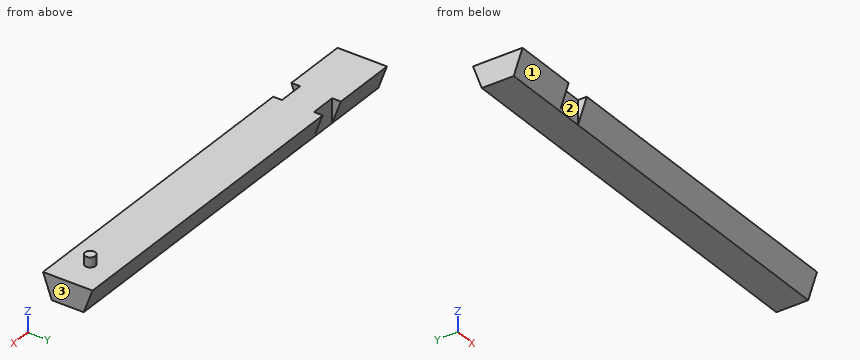
```python
from build123d import *

# Parameters (mm, degrees)
F1_DEPTH  = 203
F2_R      = 2.5
F3_DEPTH  = 10
F4_W      = 12.5
F4_H      = 4.258452
F5_DEPTH  = 11.701
F3_FACE_R = 2.5
F6_DEPTH  = 14.7


with BuildPart() as f1:
    # F0 (on Right) → F1 (new body)
    with BuildSketch(Plane.YZ):
        Polygon((-12, 11.7), (-7.741548, 0), (0, 0), (0, 11.7), align=None)
        Polygon((0, 11.7), (0, 0), (7.741548, 0), (12, 11.7), align=None)
    extrude(amount=F1_DEPTH)

    # F2 (on face) → F3 (cut)
    with BuildSketch(Plane.XY.offset(11.7)):
        with Locations((187.5, 0)):
            Circle(F2_R)
    extrude(amount=-F3_DEPTH, mode=Mode.SUBTRACT)

    # F4 (on face) → F5 (cut, through all)
    with BuildSketch(Plane.XY.offset(11.7)):
        with Locations((38.05, 9.870774)):
            Rectangle(F4_W, F4_H)
        with Locations((38.05, -9.870774)):
            Rectangle(F4_W, F4_H)
    extrude(amount=-F5_DEPTH, mode=Mode.SUBTRACT)

    # F3_face (on face) → F6 (join)
    with BuildSketch(Plane(origin=(187.5, 0, 1.7), x_dir=(1, 0, 0), z_dir=(0, 0, 1))):
        Circle(F3_FACE_R)
    extrude(amount=F6_DEPTH)


solid = f1.part
```
Source: CAD feature listing. Evaluate the final solid. Frame: model axes, mm. Face numbers are marked on the shaded views. Round coordinates to 2 decimals unless told otherwise and drop trailing zeros. Loops run counter-clockwise (first coordinate to the right, second up) from the corner with the lowest first, then second, coordinate; pieces in that order, holes last.
(1) Section query C-C (z = 7.75). Output: boundary loops of the cut face in (x, y).
From the geometry:
outline: (0, -10.56) - (31.8, -10.56) - (31.8, -7.74) - (44.3, -7.74) - (44.3, -10.56) - (203, -10.56) - (203, 10.56) - (44.3, 10.56) - (44.3, 7.74) - (31.8, 7.74) - (31.8, 10.56) - (0, 10.56) - close
(2) Section query B-B (y = 0). Output: boundary loops of the cut face in (x, z), and give its area (3 significant figures).
From the geometry:
outline: (0, 0) - (203, 0) - (203, 11.7) - (190, 11.7) - (190, 16.4) - (185, 16.4) - (185, 11.7) - (0, 11.7) - close
area: 2,400 mm2
(3) Material intervals for probe 1 along X at (y, z) = (8, 9.25); probe 2 along Y at (x, z) = (37, 4.75); probe 3 along Z at (x, y) = (14, -2), sorted ascending.
From the geometry:
probe 1: x = 0 to 31.8, 44.3 to 203
probe 2: y = -7.74 to 7.74
probe 3: z = 0 to 11.7
(4) Pull-direction query (X, two-part tool) for the marked faces 1, 2 and 3; classes: +X half, -X half, draft (parallel to the pull), parting line (faces both ways), or undercut.
From the geometry:
face 1: draft
face 2: undercut
face 3: +X half
(5) Section query D-D (x = 150). Output: boundary loops of the cut face in (y, z), and give its area (3 significant figures).
From the geometry:
outline: (-12, 11.7) - (-7.74, 0) - (7.74, 0) - (12, 11.7) - close
area: 231 mm2
(6) Contact query for flat-ended pins moving along their axis: pin 1 Ø4 at (x, z) = (100, 10) entering from -Y; pin 2 Ø12 at (x, y) = (125, -6) entering from +Z; pin 3 Ø1 at (x, z) = (106.5, 6.5) entering from +Y. Output: stop coordinate, or through.
From the geometry:
pin 1: stops at y = -12
pin 2: stops at z = 11.7
pin 3: stops at y = 10.29
(7) Section query A-A (x = 187.5). Output: boundary loops of the cut face in (y, z), and give its area (3 significant figures).
From the geometry:
outline: (-12, 11.7) - (-7.74, 0) - (7.74, 0) - (12, 11.7) - (2.5, 11.7) - (2.5, 16.4) - (-2.5, 16.4) - (-2.5, 11.7) - close
area: 254 mm2
